Input: part model. Units: mm. Frame: model coordinates. Coordinates: 2 decimals unless noted, no trailing zeros. Loops run counter-clockwise (first coordinate to the right, second up) from the corner with the lowest first, then second, coordinate; pieces in that order, holes last.
Item 1: Contact query for flat-ended pins moving along their axis: P1, Ø1.5, axis at y = -7, z = 6.5, coming from the -X side; P2, Ø1, axis at x = 0, z = 5, coming from the -Y side; P3, Ø1.5, axis at y = -2.5, z = 7.5, coming from the +X side. Output: stop coordinate, or through.
Item 2: Section A-A on y = -7.25. Return loops of the section in (x, z), and give its area (3 significant figures).
Item 3: Section B-B on z = 2.75. Return loops of the section in (x, y) (3 decimals).
Item 4: Section C-C on x = -2. Return loops of the section in (y, z).
Item 5: Section D-D on x = 0. Return loops of the section in (y, z).
Item 6: Ray query, line 1 along Y through (x, z) = (0, 6); line 2 along X through (y, z) = (-7.75, 8.25) (3 decimals); line 3 along X through (y, z) = (-5.25, 3.25). Return the intervals inside material, ascending.
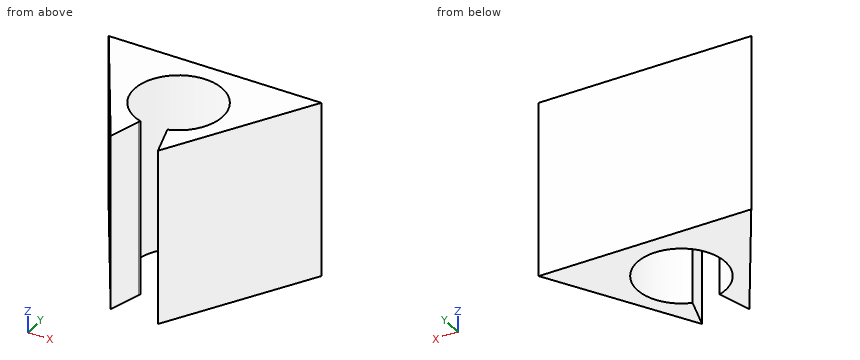
```python
from build123d import *

# Parameters (mm, degrees)
F3_DEPTH = 12.7
F4_DEPTH = 12.7
F1_R     = 3.175
F5_DEPTH = 12.7


with BuildPart() as f3:
    # F0 (on Top) → F3 (new body)
    with BuildSketch(Plane.XY):
        Polygon((0, -10.16), (0, 0), (-7.62, 0), (-1.524, -10.16), align=None)
        Polygon((7.62, 0), (0, 0), (0, -10.16), (1.524, -10.16), align=None)
    extrude(amount=F3_DEPTH)

    # F2 (on face) → F4 (cut)
    with BuildSketch(Plane.XY):
        Polygon((0, -5.08), (0, -7.62), (1.016, -7.62), (0.254, -5.08), align=None)
        Polygon((1.016, -7.62), (0, -7.62), (-1.016, -7.62), (-2.078659, -11.162197), (2.078659, -11.162197), align=None)
        Polygon((-1.016, -7.62), (0, -7.62), (0, -5.08), (-0.254, -5.08), align=None)
    extrude(amount=F4_DEPTH, mode=Mode.SUBTRACT)

    # F1 (on face) → F5 (cut)
    with BuildSketch(Plane.XY):
        with Locations((0, -4.456545)):
            Circle(F1_R)
    extrude(amount=F5_DEPTH, mode=Mode.SUBTRACT)


solid = f3.part
```
Results found:
1. P1: stops at x = -3.87
1. P2: stops at y = -1.32
1. P3: stops at x = 6.57
2. outline: (-3.27, 0) - (-1.51, 0) - (-1.51, 12.7) - (-3.27, 12.7) - close; (1.51, 0) - (3.27, 0) - (3.27, 12.7) - (1.51, 12.7) - close
2. area: 44.7 mm2
3. outline: (-7.62, 0) - (-1.693, -9.878) - (-0.974, -7.479) arc R3.175 cw (long way) to (0.974, -7.479) - (1.693, -9.878) - (7.62, 0) - close
4. outline: (-9.37, 0) - (-6.92, 0) - (-6.92, 12.7) - (-9.37, 12.7) - close; (-1.99, 0) - (0, 0) - (0, 12.7) - (-1.99, 12.7) - close
5. outline: (-1.28, 0) - (0, 0) - (0, 12.7) - (-1.28, 12.7) - close
6. line 1: y = -1.28 to 0
6. line 2: x = -2.97 to -1.055, 1.055 to 2.97
6. line 3: x = -4.47 to -3.07, 3.07 to 4.47
